```python
from build123d import *

# Parameters (mm, degrees)
SKETCH1_R           = 1.75
BOSS_EXTRUDE1_DEPTH = 4
FILLET1_R           = 3


with BuildPart() as part:
    # Sketch1 → Boss-Extrude1 (new body)
    with BuildSketch(Plane(origin=(0, 0, 0), x_dir=(1, 0, 0), z_dir=(0, 1, 0))):
        with BuildLine():
            Line((27.877501001, 2.5), (3.122498999, 2.5))
            ThreePointArc((3.122498999, 2.5), (-4, 0), (3.122498999, -2.5))
            Line((3.122498999, -2.5), (27.877501001, -2.5))
            ThreePointArc((27.877501001, -2.5), (35, 0), (27.877501001, 2.5))
        make_face()
        Circle(SKETCH1_R, mode=Mode.SUBTRACT)
        with Locations((31, 0)):
            Circle(SKETCH1_R, mode=Mode.SUBTRACT)
    extrude(amount=BOSS_EXTRUDE1_DEPTH)

    # Fillet1
    fillet1_edges = [part.edges().sort_by_distance(p)[0] for p in [
        (27.877501001, 2, 2.5),
        (3.122498999, 2, 2.5),
        (3.122498999, 2, -2.5),
        (27.877501001, 2, -2.5),
    ]]
    fillet(fillet1_edges, radius=FILLET1_R)


solid = part.part
```
Check sheet for the modelled part. Datum: model origin and axes. Units: mm. A direction names the side the tool comes from. Coordinates: 2 decimals unless noted, no trailing zeros. Order: outer loops, then holes, each group sorted by start corner. A loop starts at its lowest first (then second) coordinate and runs counter-clockwise, first axis right, second up. Notation, with made-up numbers: (-34.5, 22.5) -> (-17.5, 22.5) arc R11 ccw to (-17.5, 40.5) -> close; hole circle Ø1 at (-13.75, 60). An arc over 180 degrees is marked (long way). Write item = value, one per line. Start each with the question number.
1) Material ranges on L1, parallel to Z at x = 0, y = 2.2; L2, parallel to X at y = 2, z = 1.5; L3, parallel to X at y = 0.2, z = 1, recorded low to high.
2) Cross-section at D-D (x = 11). Enter the section's corners in (y, z).
3) Cross-section at A-A (z = 0). Enter the section's corners in (x, y), then the cut area to 3 significant figures.
4) Go/stop test with a flat-tipped pin: P1, Ø2, axis at x = 11, y = 1.5, coming from the -Z side. Record where the tip stops, or that it passes through.
5) Access from +Z, -Z, +X, -X, +Y, -Y to the whole of each face (thin tool, end or side, straight path). Record for faces 1 (the cylindrical face through (29.25, 1.97, -0.08)), 2 (the flat face through (15, 2, 2.5)), 3 (the cylindrical face through (27.64, 2.03, -2.66)).
6) Cross-section at C-C (z = 3.5). Enter the section's corners in (x, y).
7) Cross-section at B-B (x = 31). Enter the section's corners in (y, z), then the cut area to 3 significant figures.
8) Mould release check, pull along Z, two halves, no side actions. Record for faces 4 (the cylindrical face through (1.617, 1.972, 0.67)), 5 (the flat face through (15, 0, 0)), 6 (the cylindrical face through (35, 2, 0)): +Z half, -Z half, draft (parallel to the pull), parting line (faces both ways), or undercut.
Ans:
q1.L1 = -4 to -1.75, 1.75 to 4
q1.L2 = -3.71 to -0.9, 0.9 to 30.1, 31.9 to 34.71
q1.L3 = -3.87 to -1.44, 1.44 to 29.56, 32.44 to 34.87
q2.outline = (0, -2.5) -> (4, -2.5) -> (4, 2.5) -> (0, 2.5) -> close
q3.outline = (-4, 0) -> (-1.75, 0) -> (-1.75, 4) -> (-4, 4) -> close; (1.75, 0) -> (29.25, 0) -> (29.25, 4) -> (1.75, 4) -> close; (32.75, 0) -> (35, 0) -> (35, 4) -> (32.75, 4) -> close
q3.area = 128 mm²
q4.P1 = -2.5
q5.face_1 = +Y, -Y
q5.face_2 = +Z, +Y, -Y
q5.face_3 = -Z, +Y, -Y
q6.outline = (-1.94, 0) -> (1.94, 0) -> (1.94, 4) -> (-1.94, 4) -> close; (29.06, 0) -> (32.94, 0) -> (32.94, 4) -> (29.06, 4) -> close
q7.outline = (0, -4) -> (4, -4) -> (4, -1.75) -> (0, -1.75) -> close; (0, 1.75) -> (4, 1.75) -> (4, 4) -> (0, 4) -> close
q7.area = 18.0 mm²
q8.face_4 = undercut
q8.face_5 = draft
q8.face_6 = parting line
